Could you check a few things on this model? Use its own coordinates, in mm. Round coordinates to 2 decimals unless told otherwise and drop trailing zeros. Write each loop counter-clockwise with the first axis right and the second up, starting at its lowest first coordinate (ties: lowest second). Pieces come first, ordered by that corner, then holes. Notation, with made-up numbers: (53.25, -35.5) -> (60.25, -35.5) arc R27 cw to (60.25, 1.5) -> close; hole circle Ø11 at (89, 74). An arc over 180 degrees is marked (long way). Answer in a Markdown table with one row per item.
from build123d import *

# Parameters (mm, degrees)
SKETCH1_W           = 120
SKETCH1_H           = 465
BOSS_EXTRUDE1_DEPTH = 6
SKETCH4_W           = 20
SKETCH4_H           = 10
SKETCH4_W_2         = 4
SKETCH4_H_2         = 50
BOSS_EXTRUDE2_DEPTH = 6
SKETCH5_W           = 8
SKETCH5_H           = 8
CUT_EXTRUDE1_DEPTH  = 10


with BuildPart() as part:
    # Sketch1 → Boss-Extrude1 (new body)
    with BuildSketch(Plane.XY):
        Rectangle(SKETCH1_W, SKETCH1_H)
    extrude(amount=BOSS_EXTRUDE1_DEPTH)

    # Sketch4 → Boss-Extrude2 (add)
    with BuildSketch(Plane.XY.offset(6)):
        with Locations((-30, 232.5)):
            Rectangle(SKETCH4_W, SKETCH4_H)
        with Locations((0, 232.5)):
            Rectangle(SKETCH4_W, SKETCH4_H)
        with Locations((30, 232.5)):
            Rectangle(SKETCH4_W, SKETCH4_H)
        with Locations((-30, -232.5)):
            Rectangle(SKETCH4_W, SKETCH4_H)
        with Locations((0, -232.5)):
            Rectangle(SKETCH4_W, SKETCH4_H)
        with Locations((30, -232.5)):
            Rectangle(SKETCH4_W, SKETCH4_H)
        with Locations((60, 139.5)):
            Rectangle(SKETCH4_W_2, SKETCH4_H_2)
        with Locations((60, 46.5)):
            Rectangle(SKETCH4_W_2, SKETCH4_H_2)
        with Locations((60, -46.5)):
            Rectangle(SKETCH4_W_2, SKETCH4_H_2)
        with Locations((60, -139.5)):
            Rectangle(SKETCH4_W_2, SKETCH4_H_2)
    extrude(amount=-BOSS_EXTRUDE2_DEPTH)

    # Sketch5 → Cut-Extrude1 (cut)
    with BuildSketch(Plane.XY.offset(6)):
        with Locations((-56, -43.434460059)):
            Rectangle(SKETCH5_W, SKETCH5_H)
    extrude(amount=-CUT_EXTRUDE1_DEPTH, mode=Mode.SUBTRACT)


solid = part.part
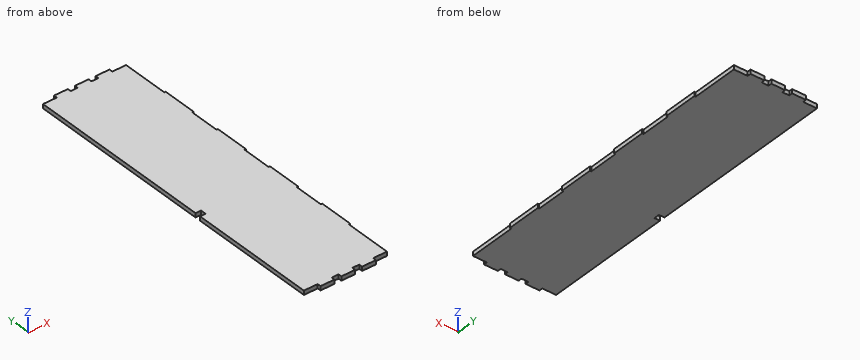
1) Imagine slicing it at A-A, the plane x = 14.5. Please give me the cut outline in (y, z), plus the area to 3 significant figures.
Findings:
| item | result |
|---|---|
| outline | (-232.5, 0) -> (232.5, 0) -> (232.5, 6) -> (-232.5, 6) -> close |
| area | 2,790 mm^2 |
2) Please list where these lines run through material, in increasing order: line 1 (Y direction, x = 14, z = 0.75); line 2 (X direction, y = 175.5, z = 5.45); line 3 (Y direction, x = -53.5, z = 5.1).
Findings:
| item | result |
|---|---|
| line 1 | y = -232.5 to 232.5 |
| line 2 | x = -60 to 60 |
| line 3 | y = -232.5 to -47.43, -39.43 to 232.5 |
3) Imagine slicing it at B-B, the plane y = -182.5. Please give me the cut outline in (x, z), plus the area to 3 significant figures.
Findings:
| item | result |
|---|---|
| outline | (-60, 0) -> (60, 0) -> (60, 6) -> (-60, 6) -> close |
| area | 720 mm^2 |
4) For pin 1 (1.8 mm diameter, centred on y = 103, z = 3.5, fed in from +X); pin 2 (1 mm diameter, centred on x = 17, z = 5, fed in from +Y); pin 3 (1.5 mm diameter, centred on y = 235.5, z = 2.5, fed in from +X), each with a flat end and sliding along its axis, tell me the tip position at first contact or that it passes through.
Findings:
| item | result |
|---|---|
| pin 1 | stops at x = 60 |
| pin 2 | stops at y = 232.5 |
| pin 3 | stops at x = 40 |
